Geometry: see drawing. Coordinates: mm, zero at the bounding-box minimum. A direction names the side the tool comes from. Coordinates: 2 decimals unless noted, no trailing zeros. Order: outer loops, then holes, each group sorted by start corner. A loop starts at its lowest first (then second) coordinate and runs counter-clockwise, first axis right, second up.
Item 1: Section D-D on z = 241.5. Return the cut outline in (x, y), then the cut area to 3 significant figures.
Item 2: Mould query, pull axis X, two halves, no side actions, for the marked faces 1, 2, 3 and 4. Classes: released by +X, released by -X, zero draft, split by the parting line, or undercut.
Item 3: Ray query, line 1 (X direction, y = 132, z = 65); line 2 (Z direction, x = 83, y = 132); line 3 (Y direction, x = 43.5, z = 132.5). Return the intervals inside material, ascending.
Item 4: Section C-C on x = 127. Return the cut outline in (y, z), then the cut area to 3 significant figures.
Item 5: Section A-A on z = 132.5. Return the cut outline in (x, y), then the cut area to 3 significant figures.
Item 6: Reachability of the marked faces 5, 6 and 7 from +Z, -Z, +X, -X, +Y, -Y: full face, straight path, thin tool, end or side. Return the list, or none.
Item 7: Section B-B on y = 132.5. State how many separate pieces and enclosed holes the cut face has, then the cut area to 3 significant figures.
Item 8: Contact query for flat-ended pins moving along their axis: P1, Ø1, axis at y = 181.5, z = 193, coming from the +X side; P2, Ø17.5, axis at y = 132.5, z = 23.5, coming from the -X side; P3, Ø5, axis at y = 238, z = 88, coming from the -X side; P4, Ø8, axis at x = 49.5, y = 153.5, coming from the -Z side. Output: stop coordinate, or through.
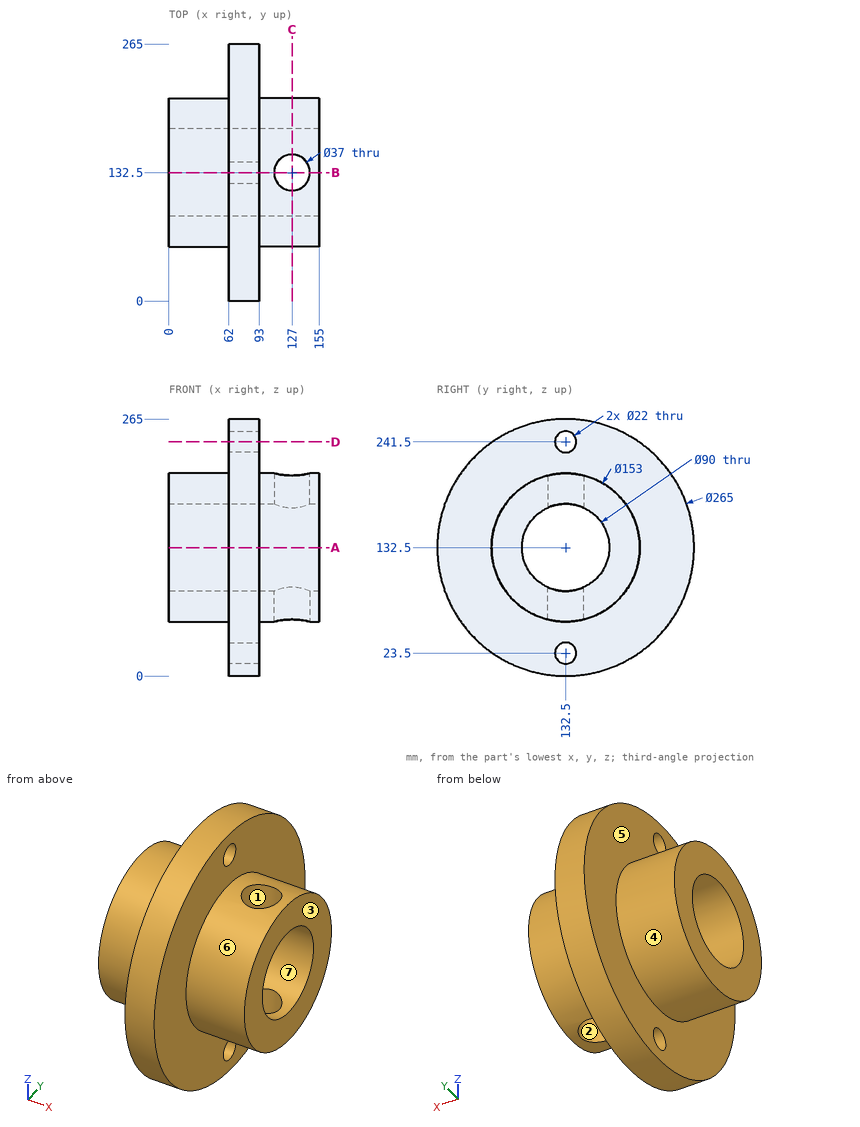
Answer list:
1. outline: (62, 57.17) - (93, 57.17) - (93, 121.5) - (62, 121.5) - close; (62, 143.5) - (93, 143.5) - (93, 207.83) - (62, 207.83) - close
1. area: 3,990 mm2
2. face 1: undercut
2. face 2: undercut
2. face 3: released by +X
2. face 4: zero draft
3. line 1: x = 0 to 108.51, 145.49 to 155
3. line 2: z = 0 to 12.51, 34.49 to 87.5, 177.5 to 230.51, 252.49 to 265
3. line 3: y = 56 to 87.5, 177.5 to 209
4. outline: (114, 58.27) - (114, 91.48) arc R45 cw to (114, 173.52) - (114, 206.73) arc R76.5 ccw to start; (151, 58.27) arc R76.5 ccw to (151, 206.73) - (151, 173.52) arc R45 cw to (151, 91.48) - close
4. area: 9,650 mm2
5. outline: (0, 56) - (62, 56) - (62, 0) - (93, 0) - (93, 56) - (155, 56) - (155, 87.5) - (0, 87.5) - close; (0, 177.5) - (155, 177.5) - (155, 209) - (93, 209) - (93, 265) - (62, 265) - (62, 209) - (0, 209) - close
5. area: 13,200 mm2
6. face 5: -X
6. face 6: +X
6. face 7: +X, -X
7. separate pieces: 6
7. enclosed holes: 0
7. area: 9,540 mm2
8. P1: stops at x = 93
8. P2: passes through
8. P3: stops at x = 62
8. P4: stops at z = 57.91
